The model under review builds one solid part; all positions refer to its coordinate system, in mm. Round coordinates to 2 decimals unless told otherwise and drop trailing zeros. Order: outer loops, then holes, each group sorted by start corner. A loop starts at its lowest first (then second) coordinate and runs counter-clockwise, first axis right, second up. Notation, with made-up numbers: M -5.75,-1 L 47.25,-1 A27 ccw 47.25,35 Z; hole C 80.25,47.25 d6. An arc over 180 degrees is marked long. Answer as a JSON object with one key per item and string values. Group by question number.
1. To check wall thickness, follow probe 1 along X at (y, z) = (0, 24); probe 2 along Z at (x, y) = (-5.5, 0.5); probe 3 along Z at (x, y) = (-64, 0.5). State the ranges of each line that lie inside material, in increasing order. Write a range as [from, to].
2. Add section B-B on y = 0.5. State the section outline as (x, z) points (1 decimal).
3. Add section A-A on z = 5.5. State the section outline as (x, y) points (1 decimal), and give its area (3 significant figures).
```python
from build123d import *

# Parameters (mm, degrees)
F1_DEPTH = 3.175


with BuildPart() as f1:
    # F0 (on Front) → F1 (new body, symmetric)
    with BuildSketch(Plane.XZ):
        with BuildLine():
            Line((-73.025, 114.3), (-128.5875, 114.3))
            Line((-128.5875, 114.3), (-128.5875, -114.3))
            Line((-128.5875, -114.3), (119.0625, -114.3))
            Line((119.0625, -114.3), (119.0625, 114.3))
            Line((119.0625, 114.3), (63.5, 114.3))
            ThreePointArc((63.5, 114.3), (62.377468, 113.835032), (61.9125, 112.7125))
            Line((61.9125, 112.7125), (61.9125, 0))
            Line((61.9125, 0), (55.5625, 0))
            Line((55.5625, 0), (55.5625, 112.7125))
            ThreePointArc((55.5625, 112.7125), (55.097532, 113.835032), (53.975, 114.3))
            Line((53.975, 114.3), (0, 114.3))
            ThreePointArc((0, 114.3), (-1.122532, 113.835032), (-1.5875, 112.7125))
            Line((-1.5875, 112.7125), (-1.5875, 0))
            Line((-1.5875, 0), (-7.9375, 0))
            Line((-7.9375, 0), (-7.9375, 112.7125))
            ThreePointArc((-7.9375, 112.7125), (-8.402468, 113.835032), (-9.525, 114.3))
            Line((-9.525, 114.3), (-63.5, 114.3))
            ThreePointArc((-63.5, 114.3), (-64.622532, 113.835032), (-65.0875, 112.7125))
            Line((-65.0875, 112.7125), (-65.0875, 0))
            Line((-65.0875, 0), (-71.4375, 0))
            Line((-71.4375, 0), (-71.4375, 112.7125))
            ThreePointArc((-71.4375, 112.7125), (-71.902468, 113.835032), (-73.025, 114.3))
        make_face()
    extrude(amount=F1_DEPTH, both=True)


solid = f1.part
```
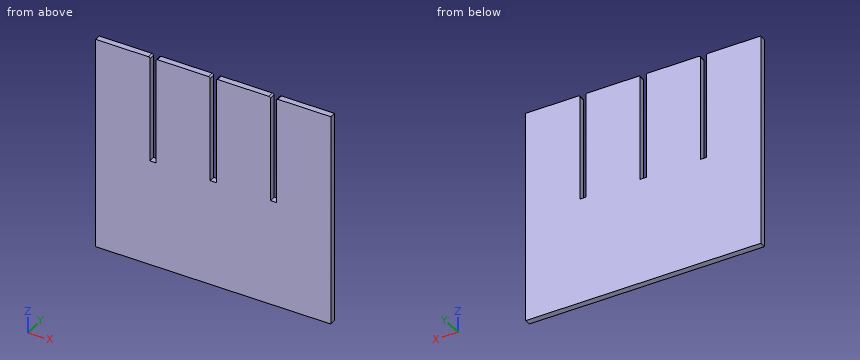
Recorded:
{
 "1": {"probe 1": "x = [-128.59, -71.44], [-65.09, -7.94], [-1.59, 55.56], [61.91, 119.06]", "probe 2": "z = [-114.3, 0]", "probe 3": "z = [-114.3, 114.22]"},
 "2": {"outline": "M -128.6,-114.3 L 119.1,-114.3 L 119.1,114.3 L 63.5,114.3 A1.6 ccw 61.9,112.7 L 61.9,0 L 55.6,0 L 55.6,112.7 A1.6 ccw 54,114.3 L 0,114.3 A1.6 ccw -1.6,112.7 L -1.6,0 L -7.9,0 L -7.9,112.7 A1.6 ccw -9.5,114.3 L -63.5,114.3 A1.6 ccw -65.1,112.7 L -65.1,0 L -71.4,0 L -71.4,112.7 A1.6 ccw -73,114.3 L -128.6,114.3 Z"},
 "3": {"outline": "M -128.6,-3.2 L -71.4,-3.2 L -71.4,3.2 L -128.6,3.2 Z; M -65.1,-3.2 L -7.9,-3.2 L -7.9,3.2 L -65.1,3.2 Z; M -1.6,-3.2 L 55.6,-3.2 L 55.6,3.2 L -1.6,3.2 Z; M 61.9,-3.2 L 119.1,-3.2 L 119.1,3.2 L 61.9,3.2 Z", "area": "1,450 mm²"}
}
